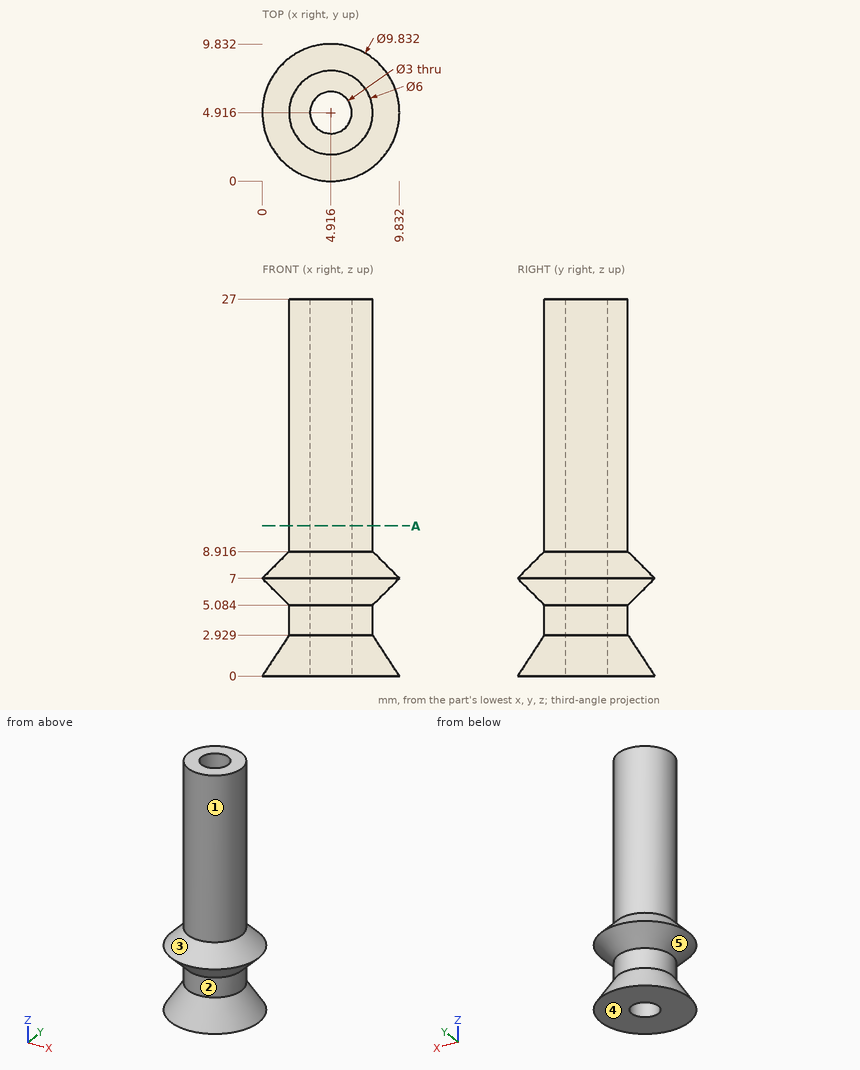
Design review of the part shown in the three views and the two pictorial views. Dimensions are in mm from the part's minimum x, y and z. A direction names the side the tool comes from. Coordinates: 2 decimals unless noted, no trailing zeros. Loops run counter-clockwise (first coordinate to the right, second up) from the corner with the lowest first, then second, coordinate; pieces in that order, holes last. Notation, with made-up numbers: (17.25, -29) -> (26.25, -29) arc R6 ccw to (26.25, -18) -> close; hole circle Ø10 at (30.25, 58.5). An arc over 180 degrees is marked (long way). Answer as CSV lines item,"result".
Item 1: Insertion check: pin 1 (1.5 mm diameter, centred on x = 7.5, z = 16.5, fed in from +Y); pin 2 (3 mm diameter, centred on x = 3, z = 17, fed in from +Y); pin 3 (5 mm diameter, centred on y = 6.5, z = 14.5, fed in from -X); pin 4 (1 mm diameter, centred on x = 4.5, y = 5.5, fed in from -Z). Each pin has a flat end and moves straight along its axis. Give the tip position at first contact, or say it passes through.
Results below:
pin 1,"stops at y = 7.29"
pin 2,"stops at y = 7.89"
pin 3,"stops at x = 1.92"
pin 4,"passes through"
Item 2: For L1, parallel to Y at x = 5, z = 25 (1 decimal); L2, parallel to X at y = 4.5, z = 10.5 (1 decimal); L3, parallel to Z at x = 7.5, y = 7 (1 decimal), list the stretches that pass through material, from the lowest coordinate up.
Results below:
L1,"y = 1.9 to 3.4, 6.4 to 7.9"
L2,"x = 1.9 to 3.5, 6.4 to 7.9"
L3,"z = 0 to 2.4, 5.4 to 8.6"
Item 3: Machinability: for the marked faces 1 and 2, which of the approach directions +Z, -Z, +X, -X, +Y, -Y give a long, thin tool a straight path to every point of the face, cutting with its end or side? Answer none if there is none.
Results below:
face 1,"+Z"
face 2,"none"
Item 4: Take a section at A-A, the plane z = 10.75. State the section outline as (x, y) points, and give its area (3 significant figures).
Results below:
outline,"circle Ø6 at (4.92, 4.92); hole circle Ø3 at (4.92, 4.92)"
area,"21.2 mm2"
Item 5: Draft analysis for pull direction Z (two halves, no side actions). For the marked faces 3, 4 and 5, state which applies: +Z half, -Z half, draft (parallel to the pull), parting line (faces both ways), or undercut.
Results below:
face 3,"+Z half"
face 4,"-Z half"
face 5,"undercut"
